```python
from build123d import *

# Parameters (mm, degrees)
F0_W     = 340
F0_H     = 1885
F1_DEPTH = 18
F2_W     = 50
F2_H     = 285
F3_DEPTH = 18
F4_W     = 18
F4_H     = 1876
F5_DEPTH = 9


with BuildPart() as f1:
    # F0 (on Front) → F1 (new body)
    with BuildSketch(Plane.XZ):
        Rectangle(F0_W, F0_H)
    extrude(amount=F1_DEPTH)

    # F2 (on face) → F3 (cut)
    with BuildSketch(Plane.XZ.offset(18)):
        with Locations((145, -800)):
            Rectangle(F2_W, F2_H)
    extrude(amount=-F3_DEPTH, mode=Mode.SUBTRACT)

    # F4 (on face) → F5 (cut)
    with BuildSketch(Plane(origin=(0, 0, 0), x_dir=(-1, 0, 0), z_dir=(0, 1, 0))):
        with Locations((-111, -4.5)):
            Rectangle(F4_W, F4_H)
    extrude(amount=-F5_DEPTH, mode=Mode.SUBTRACT)


solid = f1.part
```
Build history of the part. All positions in model axes, mm. Round coordinates to 2 decimals unless told otherwise and drop trailing zeros. Write each loop counter-clockwise with the first axis right and the second up, starting at its lowest first coordinate (ties: lowest second). Pieces come first, ordered by that corner, then holes. Notation, with made-up numbers: (-23, 23) - (21, 23) arc R28 ccw to (21, 44) - close; hole circle Ø1 at (59.5, -15.75). An arc over 180 degrees is marked (long way). Answer as CSV lines item,"result".
Q1. Drill centre lines: probe 1 along X at (y, z) = (-4.25, 557); probe 2 along Z at (x, y) = (121.5, -6); probe 3 along Z at (x, y) = (108, -7.5). Where is each one in solid material? Low to high. Write a range as [from, to].
Report:
probe 1,"x = [-170, 102], [120, 170]"
probe 2,"z = [-657.5, 942.5]"
probe 3,"z = [933.5, 942.5]"
Q2. Cut at C-C (x = 137). Write the cut outline in (y, z), and give its area (3 significant figures).
Report:
outline,"(-18, -657.5) - (0, -657.5) - (0, 942.5) - (-18, 942.5) - close"
area,"28,800 mm^2"
Q3. Cut at B-B (z = -103). Write the cut outline in (x, y), and give its area (3 significant figures).
Report:
outline,"(-170, -18) - (170, -18) - (170, 0) - (120, 0) - (120, -9) - (102, -9) - (102, 0) - (-170, 0) - close"
area,"5,960 mm^2"
Q4. Drop flat-ended pins along their axis: pin 1 (1 mm diameter, centred on x = 106.5, z = -464, fed in from +Y); pin 2 (7 mm diameter, centred on y = -11.5, z = -799, fed in from +X); pin 3 (9 mm diameter, centred on x = 154, y = -9.5, fed in from -Z). Give the stop position or say it passes through.
Report:
pin 1,"stops at y = -9"
pin 2,"stops at x = 120"
pin 3,"stops at z = -657.5"
Q5. Cut at A-A (y = -4). Write the cut outline in (x, z).
Report:
outline,"(-170, -942.5) - (102, -942.5) - (102, 933.5) - (120, 933.5) - (120, -657.5) - (170, -657.5) - (170, 942.5) - (-170, 942.5) - close"
